The model under review builds one solid part; all positions refer to its coordinate system, in mm. A direction names the side the tool comes from. Give positions to 0.01 mm unless a question says otherwise; leave off trailing zeros. Order: outer loops, then holes, each group sorted by start corner. A loop starts at its lowest first (then second) coordinate and runs counter-clockwise, first axis right, second up. Notation, with made-up numbers: (49, -17) - (92, -17) arc R13 cw to (92, -6) - close; hole circle Ø1 at (79, 0). An arc over 180 degrees is marked (long way). Answer as CSV lines item,"result". Start each with the question number.
from build123d import *

# Parameters (mm, degrees)
F0_R     = 19.05
F0_R_2   = 11.1
F1_DEPTH = 3.5
F0_R_3   = 31.75
F0_R_4   = 25.4
F2_DEPTH = 2
F3_DEPTH = 0.2
F4_R     = 2.54


with BuildPart() as f1:
    # F0 (on Top) → F1 (new body, symmetric)
    with BuildSketch(Plane.XY):
        Circle(F0_R)
        Circle(F0_R_2, mode=Mode.SUBTRACT)
    extrude(amount=F1_DEPTH, both=True)



with BuildPart() as f1b:
    # F0 (on Top) → F1, piece 2 (new body, symmetric)
    with BuildSketch(Plane.XY):
        Circle(F0_R_3)
        Circle(F0_R_4, mode=Mode.SUBTRACT)
    extrude(amount=F1_DEPTH, both=True)


with BuildPart() as f2:
    # F0 (on Top) → F2 (new body, symmetric)
    with BuildSketch(Plane.XY):
        Circle(F0_R_4)
        Circle(F0_R, mode=Mode.SUBTRACT)
    extrude(amount=F2_DEPTH, both=True)


with BuildPart() as f1_1:
    add(f1.part)

    add(f1b.part)  # F3 merges F1b

    add(f2.part)  # F3 merges F2
    # F0 (on Top) → F3 (join)
    with BuildSketch(Plane.XY):
        Circle(F0_R_4)
        Circle(F0_R, mode=Mode.SUBTRACT)
    extrude(amount=-F3_DEPTH)

    # F4
    f4_edges = [f1_1.edges().sort_by_distance(p)[0] for p in [
        (-31.75, 0, 3.5),
        (-31.75, 0, -3.5),
    ]]
    fillet(f4_edges, radius=F4_R)


solid = f1_1.part
Item 1: Take a section at A-A on x = 0. Write out the cut boundary in (y, z).
Item 2: Take a section at C-C on z = 0. Write out the cut boundary in (x, y), and give its area (3 significant figures).
Item 3: Machinability: for faces 4 (the face through (4, 19, -2)), 5 (the face through (-9, 24, -3.5)), 6 (the face through (-5.506, -24.796, 2.74)), which of the approach directions +Z, -Z, +X, -X, +Y, -Y give a long, thin tool a straight path to every point of the face, cutting with its end or side? Answer none if there is none.
Item 4: Clearance check with flat-ended pins moving along their axes: pin 1 (4 mm diameter, centred on y = 19.5, z = -2.5, fed in from -X); pin 2 (2 mm diameter, centred on y = 22, z = -2, fed in from -X); pin 3 (20 mm diameter, centred on x = 0, y = 0, fed in from -Z); pin 4 (1.5 mm diameter, centred on y = 12, z = 1, fed in from -X). State where each tip first meets the part, or that it passes through.
Item 5: For line 1 along Y through (x, z) = (-16, 2.75); line 2 along Y through (x, z) = (-9, 2.25); line 3 along Y through (x, z) = (0, 3.2), list the stretches that pass through material, from the lowest coordinate up.
Item 6: Mouldability with a two-part tool opening along Y and no side actions: class faces 1 (the face through (8, -8, -3.5)), 2 (the face through (-6.883, -30.995, 0.013)), 3 (the face through (-5.506, -24.796, -2.76)) as released by +Y, released by -Y, zero draft, split by the parting line, or undercut.
Data:
1,outline,"(-31.75, -0.96) arc R2.54 ccw to (-29.21, -3.5) - (-25.4, -3.5) - (-25.4, -2) - (-19.05, -2) - (-19.05, -3.5) - (-11.1, -3.5) - (-11.1, 3.5) - (-19.05, 3.5) - (-19.05, 2) - (-25.4, 2) - (-25.4, 3.5) - (-29.21, 3.5) arc R2.54 ccw to (-31.75, 0.96) - close; (11.1, -3.5) - (19.05, -3.5) - (19.05, -2) - (25.4, -2) - (25.4, -3.5) - (29.21, -3.5) arc R2.54 ccw to (31.75, -0.96) - (31.75, 0.96) arc R2.54 ccw to (29.21, 3.5) - (25.4, 3.5) - (25.4, 2) - (19.05, 2) - (19.05, 3.5) - (11.1, 3.5) - close"
2,outline,"circle Ø63.5 at (0, 0); hole circle Ø22.2 at (0, 0)"
2,area,"2,780 mm^2"
3,face 4,"-Z"
3,face 5,"-Z, +X, -X, +Y, -Y"
3,face 6,"+Z"
4,pin 1,"stops at x = -26.25"
4,pin 2,"stops at x = -23.63"
4,pin 3,"passes through"
4,pin 4,"stops at x = -29.69"
5,line 1,"y = -26.57 to -19.73, -10.34 to 10.34, 19.73 to 26.57"
5,line 2,"y = -30.08 to -23.75, -16.79 to -6.5, 6.5 to 16.79, 23.75 to 30.08"
5,line 3,"y = -30.41 to -25.4, -19.05 to -11.1, 11.1 to 19.05, 25.4 to 30.41"
6,face 1,"zero draft"
6,face 2,"split by the parting line"
6,face 3,"undercut"
